```python
from build123d import *

# Parameters (mm, degrees)
SKETCH1_R           = 1.5
BOSS_EXTRUDE1_DEPTH = 3


with BuildPart() as part:
    # Sketch1 → Boss-Extrude1 (new body)
    with BuildSketch(Plane(origin=(0, 0, 0), x_dir=(1, 0, 0), z_dir=(0, 1, 0))):
        with BuildLine():
            Line((-10.458743839, 9.337820174), (-7.958743839, -12.982687901))
            ThreePointArc((-7.958743839, -12.982687901), (-6.649970685, -15.519142393), (-3.983600283, -16.537453462))
            Line((-3.983600283, -16.537453462), (11.016399717, -16.537453462))
            ThreePointArc((11.016399717, -16.537453462), (13.68277012, -15.519142393), (14.991543274, -12.982687901))
            Line((14.991543274, -12.982687901), (17.491543274, 9.337820174))
            ThreePointArc((17.491543274, 9.337820174), (16.498088648, 12.449425016), (13.516399717, 13.783054613))
            Line((13.516399717, 13.783054613), (-6.483600283, 13.783054613))
            ThreePointArc((-6.483600283, 13.783054613), (-9.465289213, 12.449425016), (-10.458743839, 9.337820174))
        make_face()
        with Locations((-3.983600283, -12.537453462)):
            Circle(SKETCH1_R, mode=Mode.SUBTRACT)
        with Locations((11.016399717, -12.537453462)):
            Circle(SKETCH1_R, mode=Mode.SUBTRACT)
        with Locations((3.516399717, -7.537453462)):
            Circle(SKETCH1_R, mode=Mode.SUBTRACT)
        with Locations((11.016399717, -2.537453462)):
            Circle(SKETCH1_R, mode=Mode.SUBTRACT)
        with Locations((-3.983600283, -2.537453462)):
            Circle(SKETCH1_R, mode=Mode.SUBTRACT)
        with Locations((13.516399717, 9.783054613)):
            Circle(SKETCH1_R, mode=Mode.SUBTRACT)
        with Locations((-6.483600283, 9.783054613)):
            Circle(SKETCH1_R, mode=Mode.SUBTRACT)
    extrude(amount=BOSS_EXTRUDE1_DEPTH)


solid = part.part
```
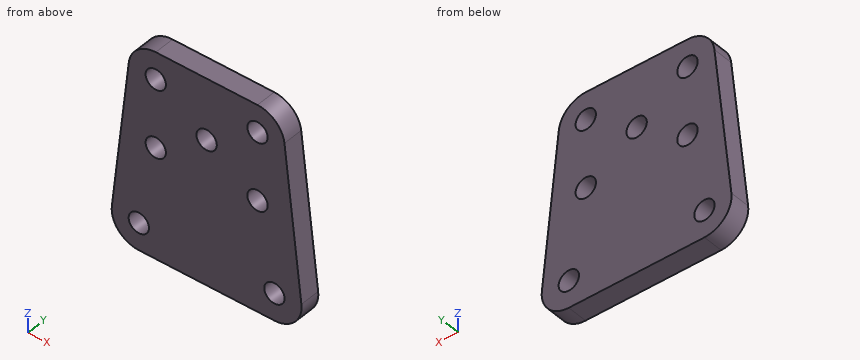
Check sheet for the modelled part. Datum: model origin and axes. Units: mm. Coordinates: 2 decimals unless noted, no trailing zeros. Order: outer loops, then holes, each group sorted by start corner. A loop starts at its lowest first (then second) coordinate and runs counter-clockwise, first axis right, second up. Notation, with made-up numbers: (75, -29.75) -> (125, -29.75) arc R10 ccw to (125, -25.75) -> close; hole circle Ø3 at (37, 3.5). An arc over 180 degrees is marked (long way). Write item = value, one per line. Start each with the question number.
1) Material ranges on L1, parallel to X at y = 2.85, z = -10; L2, parallel to X at y = 0.3, z = -8.5; L3, parallel to Z at x = -3.75, y = 0.8, recorded low to high.
2) Cross-section at D-D (y = 1.75). Enter the section's corners in (x, z).
3) Cross-section at C-C (x = 4.25). Enter the section's corners in (y, z), then the cut area to 3 significant figures.
4) Go/stop test with a flat-tipped pin: P1, Ø1.8, axis at x = -6.48, z = -9.78, coming from the -Y side. Record where the tip stops, or that it passes through.
5) Cross-section at A-A (x = -4.5). Enter the section's corners in (y, z), then the cut area to 3 significant figures.
6) Cross-section at B-B (z = 12). Enter the section's corners in (x, y).
Ans:
q1.L1 = -10.48 to -7.97, -5 to 12.03, 15 to 17.51
q1.L2 = -10.36 to -7.26, -5.71 to 12.74, 14.29 to 17.4
q1.L3 = -13.78 to 1.06, 4.02 to 11.06, 14.02 to 16.54
q2.outline = (-10.46, -9.34) arc R4 ccw to (-6.48, -13.78) -> (13.52, -13.78) arc R4 ccw to (17.49, -9.34) -> (14.99, 12.98) arc R4 ccw to (11.02, 16.54) -> (-3.98, 16.54) arc R4 ccw to (-7.96, 12.98) -> close; hole circle Ø3 at (-6.48, -9.78); hole circle Ø3 at (-3.98, 2.54); hole circle Ø3 at (-3.98, 12.54); hole circle Ø3 at (3.52, 7.54); hole circle Ø3 at (11.02, 2.54); hole circle Ø3 at (11.02, 12.54); hole circle Ø3 at (13.52, -9.78)
q3.outline = (0, -13.78) -> (3, -13.78) -> (3, 6.23) -> (0, 6.23) -> close; (0, 8.85) -> (3, 8.85) -> (3, 16.54) -> (0, 16.54) -> close
q3.area = 83.1 mm²
q4.P1 = through
q5.outline = (0, -13.78) -> (3, -13.78) -> (3, 1.13) -> (0, 1.13) -> close; (0, 3.95) -> (3, 3.95) -> (3, 11.13) -> (0, 11.13) -> close; (0, 13.95) -> (3, 13.95) -> (3, 16.5) -> (0, 16.5) -> close
q5.area = 74.0 mm²
q6.outline = (-8.07, 0) -> (-5.38, 0) -> (-5.38, 3) -> (-8.07, 3) -> close; (-2.58, 0) -> (9.62, 0) -> (9.62, 3) -> (-2.58, 3) -> close; (12.42, 0) -> (15.1, 0) -> (15.1, 3) -> (12.42, 3) -> close
